Source: CAD feature listing. Evaluate the final solid. Frame: model axes, mm. A direction names the side the tool comes from. Give positions to 0.01 mm unless a question says otherwise; leave off trailing zeros. Loops run counter-clockwise (first coordinate to the right, second up) from the corner with the lowest first, then second, coordinate; pieces in that order, holes last. Notation, with made-up numbers: M 86,21 L 114,21 A11 ccw 114,40 Z; hole C 89,8.25 d5. An arc over 180 degrees is marked long. Write item = value, one per line.
from build123d import *

# Parameters (mm, degrees)
SKETCH1_W           = 273.05
SKETCH1_H           = 215.9
BOSS_EXTRUDE1_DEPTH = 19.05
FILLET1_R           = 9.525
CUT_EXTRUDE1_DEPTH  = 12.7


with BuildPart() as part:
    # Sketch1 → Boss-Extrude1 (new body)
    with BuildSketch(Plane(origin=(0, 0, 0), x_dir=(1, 0, 0), z_dir=(0, 1, 0))):
        with Locations((136.525, 107.95)):
            Rectangle(SKETCH1_W, SKETCH1_H)
    extrude(amount=BOSS_EXTRUDE1_DEPTH)

    # Fillet1
    fillet1_edges = [part.edges().sort_by_distance(p)[0] for p in [
        (0, 9.525, -215.9),
        (273.05, 9.525, -215.9),
        (273.05, 9.525, 0),
        (0, 9.525, 0),
    ]]
    fillet(fillet1_edges, radius=FILLET1_R)

    # Sketch3 → Cut-Extrude1 (cut)
    with BuildSketch(Plane(origin=(0, 19.05, 0), x_dir=(1, 0, 0), z_dir=(0, 1, 0))):
        with BuildLine():
            Line((269.875, 9.525), (269.875, 206.375))
            ThreePointArc((269.875, 206.375), (268.015128061, 210.865128061), (263.525, 212.725))
            Line((263.525, 212.725), (9.525, 212.725))
            ThreePointArc((9.525, 212.725), (5.034871939, 210.865128061), (3.175, 206.375))
            Line((3.175, 206.375), (3.175, 9.525))
            ThreePointArc((3.175, 9.525), (5.034871939, 5.034871939), (9.525, 3.175))
            Line((9.525, 3.175), (263.525, 3.175))
            ThreePointArc((263.525, 3.175), (268.015128061, 5.034871939), (269.875, 9.525))
        make_face()
    extrude(amount=-CUT_EXTRUDE1_DEPTH, mode=Mode.SUBTRACT)


solid = part.part
1. Reachability of faces 4 (the cylindrical face through (2.72, 9.66, -213.04)), 5 (the flat face through (269.875, 13, -107)) from +Z, -Z, +X, -X, +Y, -Y: full face, straight path, thin tool, end or side. Return the list, or none.
Derived:
face_4 = -Z, -X, +Y, -Y
face_5 = +Y
2. Cut plane B-B, the plane x = 21.5. Return the cut outline in (y, z) (3 decimals).
Derived:
outline = M 0,-215.9 L 19.05,-215.9 L 19.05,-212.725 L 6.35,-212.725 L 6.35,-3.175 L 19.05,-3.175 L 19.05,0 L 0,0 Z
3. Cut plane C-C, the plane z = -133. Return the cut outline in (x, y) (3 decimals).
Derived:
outline = M 0,0 L 273.05,0 L 273.05,19.05 L 269.875,19.05 L 269.875,6.35 L 3.175,6.35 L 3.175,19.05 L 0,19.05 Z
4. Cut plane A-A, the plane y = 9.5. Return the cut outline in (x, z) (3 decimals), then the cut area to 3 significant figures.
Derived:
outline = M 0,-206.375 A9.525 ccw 9.525,-215.9 L 263.525,-215.9 A9.525 ccw 273.05,-206.375 L 273.05,-9.525 A9.525 ccw 263.525,0 L 9.525,0 A9.525 ccw 0,-9.525 Z; hole M 3.175,-206.375 A6.35 ccw 9.525,-212.725 L 263.525,-212.725 A6.35 ccw 269.875,-206.375 L 269.875,-9.525 A6.35 ccw 263.525,-3.175 L 9.525,-3.175 A6.35 ccw 3.175,-9.525 Z
area = 3,020 mm²
5. First-contact query: pin 1 Ø10 at (x, z) = (152, -131.5) entering from +Y. Flat tip, straight axial feed; report the tip coordinate or a pass-through.
Derived:
pin_1 = 6.35
6. Pull-direction query (Z, two-part tool) for faces 1 (the flat face through (0, 9, -107)), 2 (the cylindrical face through (268.06, 12.79, -210.82)), 3 (the cylindrical face through (270.19, 9.66, -2.72)); classes: +Z half, -Z half, draft (parallel to the pull), parting line (faces both ways), or undercut.
Derived:
face_1 = draft
face_2 = undercut
face_3 = +Z half
7. Material intervals for probe 1 along Z at (x, y) = (145, 12.75) (3 decimals); probe 2 along X at (y, z) = (18.25, -204) (3 decimals); probe 3 along Y at (x, z) = (173, -130.5), sorted ascending. Write a range as from..to.
Derived:
probe_1 = -215.9..-212.725, -3.175..0
probe_2 = 0..3.175, 269.875..273.05
probe_3 = 0..6.35
